```python
from build123d import *

# Parameters (mm, degrees)
BOSS_EXTRUDE1_DEPTH = 125
SKETCH3_R           = 0.9
CUT_EXTRUDE1_DEPTH  = 277.372809806
CHAMFER1_SIZE       = 1
CHAMFER2_SIZE       = 1
CUT_EXTRUDE2_REACH  = 278.373
SKETCH4_W           = 18
SKETCH4_H           = 14


with BuildPart() as part:
    # Sketch1 → Boss-Extrude1 (new, symmetric)
    with BuildSketch(Plane.XY):
        with BuildLine():
            Line((-75.1, 0), (-75.1, 115.2))
            ThreePointArc((-75.1, 115.2), (0, 190.3), (75.1, 115.2))
            Line((75.1, 115.2), (75.1, 0))
            Line((75.1, 0), (77.1, 0))
            Line((77.1, 0), (77.1, 115.2))
            ThreePointArc((77.1, 115.2), (0, 192.3), (-77.1, 115.2))
            Line((-77.1, 115.2), (-77.1, 0))
            Line((-77.1, 0), (-75.1, 0))
        make_face()
    extrude(amount=BOSS_EXTRUDE1_DEPTH, both=True)

    # Sketch3 → Cut-Extrude1 (cut, through all)
    with BuildSketch(Plane.ZY.offset(77.1)):
        with Locations((-115, 15)):
            Circle(SKETCH3_R)
        with Locations((-75, 15)):
            Circle(SKETCH3_R)
        with Locations((-35, 15)):
            Circle(SKETCH3_R)
        with Locations((-115, 45)):
            Circle(SKETCH3_R)
    cut_extrude1 = extrude(amount=-CUT_EXTRUDE1_DEPTH, mode=Mode.SUBTRACT)

    # Mirror1: Cut-Extrude1 across plane
    add(cut_extrude1.mirror(Plane.XY), mode=Mode.SUBTRACT)

    # Chamfer1
    chamfer1_edges = [part.edges().sort_by_distance(p)[0] for p in [
        (-77.1, 45, -115.9),
        (-77.1, 15, -35.9),
        (-77.1, 15, -75.9),
        (-77.1, 15, -115.9),
        (-77.1, 45, 115.9),
        (-77.1, 15, 35.9),
        (-77.1, 15, 75.9),
        (-77.1, 15, 115.9),
        (-75.1, 15, 115.9),
    ]]
    chamfer(chamfer1_edges, length=CHAMFER1_SIZE - 0.0001)  # a hair under: the kernel refuses the full size

    # Chamfer2
    chamfer2_edges = [part.edges().sort_by_distance(p)[0] for p in [
        (77.1, 45, -115.9),
        (77.1, 15, -35.9),
        (77.1, 15, -75.9),
        (77.1, 15, -115.9),
        (77.1, 45, 115.9),
        (77.1, 15, 35.9),
        (77.1, 15, 75.9),
        (77.1, 15, 115.9),
    ]]
    chamfer(chamfer2_edges, length=CHAMFER2_SIZE)

    # Sketch4 → Cut-Extrude2 (cut, up to next)
    with BuildSketch(Plane.ZY.offset(77.1), mode=Mode.PRIVATE) as cut_extrude2_sk1:
        with Locations((-20, 77)):
            Rectangle(SKETCH4_W, SKETCH4_H)
    cut_extrude2_tool1 = extrude(cut_extrude2_sk1.sketch, amount=-CUT_EXTRUDE2_REACH, mode=Mode.PRIVATE) & part.part
    add(cut_extrude2_tool1.solids().sort_by_distance((-77.1, 77, -20))[0], mode=Mode.SUBTRACT)


solid = part.part
```
Verification items for the finished model (mm, model axes). Give positions to 0.01 mm unless a question says otherwise; leave off trailing zeros. Order: outer loops, then holes, each group sorted by start corner. A loop starts at its lowest first (then second) coordinate and runs counter-clockwise, first axis right, second up. Notation, with made-up numbers: (22.25, 47) - (72.25, 47) arc R27 cw to (72.25, 80) - close; hole circle Ø4 at (60.5, 55). An arc over 180 degrees is marked (long way). Answer as CSV lines item,"result". Start each with the question number.
Item 1: Gauge pin test, flat ends, axial feed: pin 1 (8 mm diameter, centred on x = 21.5, z = 78.5, fed in from -Y); pin 2 (5 mm diameter, centred on x = -29.5, z = -24.5, fed in from +Y); pin 3 (2 mm diameter, centred on y = 15, z = 115, fed in from -X); pin 4 (1.1 mm diameter, centred on y = 15, z = 115, fed in from -X). Record the tip position at first contact, or that the pin passes through.
Item 2: Section check C-C, the plane y = 74. Record the boundary of the cut face in (x, z).
Item 3: Mould release check, pull along X, two halves, no side actions. Record for faces 1 (the face through (77.1, 57, 2)), 2 (the face through (-75.1, 57, 2)), 3 (the face through (-77.1, 58, 2)), 4 (the face through (1.7, 192.28, 1.75)): released by +X, released by -X, zero draft, split by the parting line, or undercut.
Item 4: Section check D-D, the plane x = 0. Record the boundary of the cut face in (y, z).
Item 5: Material ranges on L1, parallel to X at y = 38, z = -36; L2, parallel to Z at x = 75.3, y = 45; L3, parallel to X at y = 156, z = -101, recorded low to high.
Item 6: Section check B-B, the plane y = 24.5. Record the boundary of the cut face in (x, z), plus the area to 3 significant figures.
Item 7: Section check A-A, the plane z = -23. Record the boundary of the cut face in (x, y).
Filled in:
1,pin 1,"y = 185.84"
1,pin 2,"y = 187.42"
1,pin 3,"x = -76.2"
1,pin 4,"through"
2,outline,"(-77.1, -125) - (-75.1, -125) - (-75.1, -29) - (-77.1, -29) - close; (-77.1, -11) - (-75.1, -11) - (-75.1, 125) - (-77.1, 125) - close; (75.1, -125) - (77.1, -125) - (77.1, 125) - (75.1, 125) - close"
3,face 1,"released by +X"
3,face 2,"undercut"
3,face 3,"released by -X"
3,face 4,"split by the parting line"
4,outline,"(190.3, -125) - (192.3, -125) - (192.3, 125) - (190.3, 125) - close"
5,L1,"-77.1 to -75.1, 75.1 to 77.1"
5,L2,"-125 to -115.9, -114.1 to 114.1, 115.9 to 125"
5,L3,"-65.42 to -63.05, 63.05 to 65.42"
6,outline,"(-77.1, -125) - (-75.1, -125) - (-75.1, 125) - (-77.1, 125) - close; (75.1, -125) - (77.1, -125) - (77.1, 125) - (75.1, 125) - close"
6,area,"1,000 mm^2"
7,outline,"(-77.1, 0) - (-75.1, 0) - (-75.1, 70) - (-77.1, 70) - close; (-77.1, 84) - (-75.1, 84) - (-75.1, 115.2) arc R75.1 cw to (75.1, 115.2) - (75.1, 0) - (77.1, 0) - (77.1, 115.2) arc R77.1 ccw to (-77.1, 115.2) - close"
